CAD build for the part. Positions are in the model's coordinates, mm. A direction names the side the tool comes from. Give positions to 0.01 mm unless a question says otherwise; leave off trailing zeros. Loops run counter-clockwise (first coordinate to the right, second up) from the corner with the lowest first, then second, coordinate; pieces in that order, holes last.
Item 1: Mould opens along Y. For faces 3 (the flat face through (30.7, -20.4, 4.9)), 4 (the cylindrical face through (47.244, -6.972, 4.93)), 5 (the flat face through (35.675, 10.38, 4.93)) say: released by +Y, released by -Y, zero draft, split by the parting line, or undercut.
Item 2: Probe probe 1 along X at (y, z) = (-3, 4); probe 2 along X at (y, z) = (-11, 4); probe 3 along Y at (x, z) = (0, 5.75). List the from-to ranges inside material, lowest first.
Item 3: Saw through at B-B on x = -44. Give the cut face in (y, z).
Item 4: Saw through at A-A on y = -11.5. Give the cut face in (x, z), plus the area to 4 significant figures.
Item 5: Which spindle directions (+Z, -Z, +X, -X, +Y, -Y) get a long thin tool onto all of the face, cutting with end or side? Do faces 1 (the cylindrical face through (22.307, -17.013, 4.93)), 2 (the flat face through (-1, -2, 0)). Say none if no direction does.
Item 6: Saw through at C-C on z = 2. Give the cut face in (x, y), plus the area to 3 significant figures.
Item 7: Saw through at D-D on y = -3.5. Give the cut face in (x, z).
Item 8: Drop flat-ended pins along their axis: P1, Ø2, axis at x = 38.5, z = 7, coming from the +Y side; P2, Ø1, axis at x = -30, z = 4, coming from the +Y side; P3, Ø2, axis at y = 5.5, z = 8.5, coming from the +X side. Give the stop position or say it passes through.
from build123d import *

# Parameters (mm, degrees)
SKETCH1_R           = 7.775663032
BOSS_EXTRUDE1_DEPTH = 10


with BuildPart() as part:
    # Sketch1 → Boss-Extrude1 (new body)
    with BuildSketch(Plane.XY):
        with BuildLine():
            Line((0, 19.052140157), (21.399532491, 19.052140157))
            ThreePointArc((21.399532491, 19.052140157), (22.771528747, 18.846885641), (24.023387185, 18.249095047))
            Line((24.023387185, 18.249095047), (47.657624277, 2.287166265))
            ThreePointArc((47.657624277, 2.287166265), (51.92269033, -16.338565843), (33.626657752, -21.848908566))
            Line((33.626657752, -21.848908566), (27.605393149, -18.872072273))
            ThreePointArc((27.605393149, -18.872072273), (22.228507675, -16.996447441), (16.556211898, -16.492536209))
            Line((16.556211898, -16.492536209), (0, -17.070741143))
            Line((0, -17.070741143), (0, 0))
            Line((0, 0), (0, 19.052140157))
        make_face()
        with Locations((39.827165888, -9.307103614)):
            Circle(SKETCH1_R, mode=Mode.SUBTRACT)
    boss_extrude1 = extrude(amount=BOSS_EXTRUDE1_DEPTH)

    # Mirror1: Boss-Extrude1 across plane
    add(boss_extrude1.mirror(Plane(origin=(0, 0, 10), x_dir=(0, 0, 1), z_dir=(1, 0, 0))))


solid = part.part
Results below:
1. face 3: released by -Y
1. face 4: undercut
1. face 5: released by +Y
2. probe 1: x = -52.32 to -44.37, -35.28 to 35.28, 44.37 to 52.32
2. probe 2: x = -53.72 to -47.42, -32.24 to 32.24, 47.42 to 53.72
2. probe 3: y = -17.07 to 19.05
3. outline: (-22.66, 0) - (-15.87, 0) - (-15.87, 10) - (-22.66, 10) - close; (-2.75, 0) - (4.76, 0) - (4.76, 10) - (-2.75, 10) - close
4. outline: (-53.65, 0) - (-47.29, 0) - (-47.29, 10) - (-53.65, 10) - close; (-32.37, 0) - (32.37, 0) - (32.37, 10) - (-32.37, 10) - close; (47.29, 0) - (53.65, 0) - (53.65, 10) - (47.29, 10) - close
4. area: 774.5 mm2
5. face 1: +Z, -Z, -Y
5. face 2: -Z, +X, -X, +Y, -Y
6. outline: (-47.66, 2.29) arc R13.99 ccw to (-33.63, -21.85) - (-27.61, -18.87) arc R23.11 cw to (-16.56, -16.49) - (0, -17.07) - (16.56, -16.49) arc R23.11 cw to (27.61, -18.87) - (33.63, -21.85) arc R13.99 ccw to (47.66, 2.29) - (24.02, 18.25) arc R4.69 ccw to (21.4, 19.05) - (-21.4, 19.05) arc R4.69 ccw to (-24.02, 18.25) - close; hole circle Ø15.55 at (-39.83, -9.31); hole circle Ø15.55 at (39.83, -9.31)
6. area: 3,040 mm2
7. outline: (-52.56, 0) - (-45, 0) - (-45, 10) - (-52.56, 10) - close; (-34.66, 0) - (34.66, 0) - (34.66, 10) - (-34.66, 10) - close; (45, 0) - (52.56, 0) - (52.56, 10) - (45, 10) - close
8. P1: stops at y = 9.15
8. P2: stops at y = 14.55
8. P3: stops at x = 44.38
